The listing builds one solid part. Answer for the finished solid, in the listing's coordinates (mm). Face numbers are marked on the shaded views. Coordinates: 2 decimals unless noted, no trailing zeros. Write each loop counter-clockwise with the first axis right and the second up, starting at its lowest first coordinate (ties: lowest second). Pieces come first, ordered by that corner, then holes. Notation, with made-up numbers: M 48.5,45.5 L 97.5,45.5 A12 cw 97.5,53.5 Z; hole C -28,37 d11. An arc over 180 degrees is marked long. Answer as CSV lines item,"result". Start each with the question number.
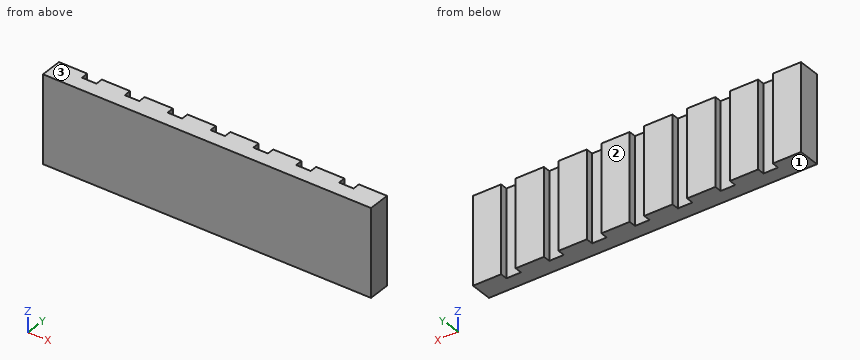
```python
from build123d import *

# Parameters (mm, degrees)
F0_W     = 38.1
F0_H     = 152.4
F1_DEPTH = 285.75
F2_W     = 25.4
F2_H     = 12.7
F3_DEPTH = 152.401


with BuildPart() as f1:
    # F0 (on Right) → F1 (new body, symmetric)
    with BuildSketch(Plane.YZ):
        Rectangle(F0_W, F0_H)
    extrude(amount=F1_DEPTH, both=True)

    # F2 (on face) → F3 (cut, through all)
    with BuildSketch(Plane.XY.offset(76.2)):
        with Locations((-223.80575, 12.7)):
            Rectangle(F2_W, F2_H)
        with Locations((-149.1615, 12.7)):
            Rectangle(F2_W, F2_H)
        with Locations((-74.51725, 12.7)):
            Rectangle(F2_W, F2_H)
        with Locations((0.127, 12.7)):
            Rectangle(F2_W, F2_H)
        with Locations((74.77125, 12.7)):
            Rectangle(F2_W, F2_H)
        with Locations((149.4155, 12.7)):
            Rectangle(F2_W, F2_H)
        with Locations((224.05975, 12.7)):
            Rectangle(F2_W, F2_H)
    extrude(amount=-F3_DEPTH, mode=Mode.SUBTRACT)


solid = f1.part
```
1) Find the intervals of material crossed by line 1 (Y direction, x = -3, z = 33.5), in increasing order. Write a range as from..to.
2) For a pull along Z with two mould halves and no side action, classify the marked faces 1, 2 and 3 as +Z half, -Z half, draft (parallel to the pull), parting line (faces both ways), or undercut.
3) This flat-tipped pin is pushed along its axis until it touches: P1, Ø4, axis at x = -215.5, z = -27.5, coming from the +Y side. Where does it stop, or does it pass through?
4) The part is cut by section B-B (x = -144). Determine the outline of the cut face in (y, z), then the cut area to 3 significant figures.
Completed:
1,line 1,"-19.05..6.35"
2,face 1,"-Z half"
2,face 2,"draft"
2,face 3,"+Z half"
3,P1,"y = 6.35"
4,outline,"M -19.05,-76.2 L 6.35,-76.2 L 6.35,76.2 L -19.05,76.2 Z"
4,area,"3,870 mm²"
